Build history of the part. All positions in model axes, mm. Face numbers are marked on the shaded views. A direction names the side the tool comes from. Round coordinates to 2 decimals unless told otherwise and drop trailing zeros. Write each loop counter-clockwise with the first axis right and the second up, starting at its lowest first coordinate (ties: lowest second). Pieces come first, ordered by that corner, then holes. Notation, with made-up numbers: M 6,75 L 21,75 A19 cw 21,101 Z; hole C 43,51.5 d5. An arc over 180 degrees is marked long. Write item = value, one per line. Start each with the question number.
Q1. Drop flat-ended pins along their axis: P1, Ø10, axis at x = -36, z = 11, coming from the -Y side; P2, Ø16, axis at x = -37.5, z = 17, coming from the +Y side; P3, Ø3, axis at y = 9.5, z = 31.5, coming from the +X side; P4, Ø3, axis at y = 14, z = 18.5, coming from the -X side. Give the stop position or say it passes through.
Q2. Pull direction X, two halves, no side cores. Call the marked faces 6, 7 and 8: released by +X, released by -X, zero draft, split by the parting line, or undercut.
Q3. Band-saw the part on C-C on y = 29. Write the cut outline in (x, z).
Q4. Band-saw the part on B-B on x = -9.25. Write the cut outline in (y, z).
Q5. Probe L1, parallel to Y at x = -9, z = 2; L2, parallel to X at y = 11, z = 1.8; L3, parallel to Y at x = 14.5, z = 0.8. List the from-to ranges inside material, lowest first.
Q6. Tool access for the marked faces 1, 2, 3, 4 and 5: list every direction of +Z, -Z, +X, -X, +Y, -Y with a clear straight run to the whole face (end or side of a thin tool).
Q7. Band-saw the part on A-A on y = 9.5. Write the cut outline in (x, z), plus the area to 3 significant figures.
Q8. Band-saw the part on D-D on z = 13. Write the cut outline in (x, y), plus the area to 3 significant figures.
Autodesk Fusion 360 part; units mm, degrees
sketch "Szkic1" plane through (0, 0, 0) normal (0, 0, 1) x (1, 0, 0)
  line L0 (-20, 15) -> (1.5, 15)
  line L1 (1.5, 15) -> (1.5, 5)
  line L2 (1.5, 5) -> (-20, 5)
  line L3 (-20, 5) -> (-20, 15)
  line L4 (-23, 18) -> (4.5, 18)
  line L5 (4.5, 18) -> (4.5, 2)
  line L6 (4.5, 2) -> (-23, 2)
  line L7 (-23, 2) -> (-23, 18)
  line L8 (-43, 18) -> (24.5, 18)
  line L9 (24.5, 18) -> (24.5, 2)
  line L10 (24.5, 2) -> (-43, 2)
  line L11 (-43, 2) -> (-43, 18)
  line L12 (-23, 18) -> (4, 18)
  line L13 (4, 18) -> (4, 38)
  line L14 (4, 38) -> (-23, 38)
  line L15 (-23, 38) -> (-23, 18)
  dimension "d1" = 21.5
  dimension "d2" = 10
  dimension "d3" = 3
  dimension "d4" = 3
  dimension "d5" = 3
  dimension "d6" = 3
  dimension "d7" = 20
  dimension "d8" = 20
extrude "Wyciągnięcie proste4" add sketch "Szkic1" along normal blind 3 contours L4 L8 L12 L13 L14 L15 | L7 L8 L10 L11 | L5 L8 L9 L10 makes body 1 at (-36.3333, 12.6667, 0) makes body 2 at (17.8333, 7.3333, 0)
extrude "Wyciągnięcie proste5" add sketch "Szkic1" along normal blind 30 contours L4 L5 L6 L7 L8 L10 L12 bodies 1 2
extrude "Extrude6" add 1 faces at (-12.8333, 3, 30) along direction (0, 0, 1) blind 10 on bodies 1 bodies 1
extrude "Extrude7" add 1 faces at (-12.8333, 3, 40) along direction (0, 0, 1) blind 3 on bodies 1 bodies 1
sketch "Sketch2" plane through (0, 0, 0) normal (0, 1, 0) x (1, 0, 0)
  line L0 (-43, -3) -> (-23, -23)
  line L1 (-23, -23) -> (-23, -3)
  line L2 (-23, -3) -> (-43, -3)
  line L3 (24.5, -3) -> (4.5, -23)
  line L4 (4.5, -23) -> (4.5, -3)
  line L5 (4.5, -3) -> (24.5, -3)
  dimension "d23" = 135
extrude "Extrude8" add sketch "Sketch2" along normal blind 2 from surface at 2 contours L0 L1 L2 bodies 1
extrude "Extrude9" add sketch "Sketch2" along normal blind 2 from surface at 2 contours L3 L4 L5 bodies 1
extrude "Extrude10" add 1 faces at (4, 24.6667, 1) along direction (1, 0, 0) blind 0.5 on bodies 1 bodies 1
extrude "Extrude11" add 1 faces at (11.1667, 18, 1) along direction (0, 1, 0) blind 2 on bodies 1 bodies 1
extrude "Extrude12" add sketch "Sketch2" along normal blind 2 from surface at 18 contours L3 L4 L5 bodies 1
extrude "Extrude13" add sketch "Sketch2" along normal blind 2 from surface at 18 separate body contours L0 L1 L2 makes body 3
extrude "Extrude14" add 1 faces at (-36.3333, 18, 1) along direction (0, 1, 0) blind 2 on bodies 1 bodies 1 3
extrude "Extrude15" add 1 faces at (-13.8333, 18, 16.3333) along direction (0, 1, 0) blind 2 on bodies 1 bodies 1
sketch "Sketch3" plane through (4.5, 0, 0) normal (1, 0, 0) x (0, 1, 0)
  line L0 (20, 3) -> (20, 0)
  line L1 (20, 0) -> (38, 0)
  line L2 (38, 0) -> (38, 3)
  line L3 (38, 3) -> (20, 3)
  line L4 (20, 23) -> (38, 3)
  line L5 (20, 3) -> (20, 23)
sketch "Sketch4" plane through (-23, 0, 0) normal (-1, 0, 0) x (0, -1, 0)
  line L0 (-20, 0) -> (-20, 3)
  line L1 (-20, 3) -> (-38, 3)
  line L2 (-38, 3) -> (-38, 0)
  line L3 (-38, 0) -> (-20, 0)
  line L4 (-38, 3) -> (-20, 3)
  line L5 (-20, 23) -> (-38, 3)
  line L6 (-20, 23) -> (-20, 3)
extrude "Extrude16" add sketch "Sketch3" against normal blind 2 contours L3 L4 L5 bodies 1
extrude "Extrude17" add sketch "Sketch4" against normal blind 2 contours L1 L4 L5 L6 bodies 1
sketch "Sketch5" plane through (0, 0, 3) normal (0, 0, 1) x (-1, 0, 0)
  line L0 (-24.5, -18) -> (-4.5, -18)
  line L1 (-4.5, -18) -> (-4.5, -4)
  line L2 (-4.5, -4) -> (-24.5, -4)
  line L3 (-24.5, -4) -> (-24.5, -18)
  circle A0 centre (-14.5, -11) radius 2.5
  circle A1 centre (33, -11) radius 2.5
  line L4 (23, -2) -> (23, -20)
  circle A2 centre (9.25, -29) radius 2.5
  line L5 (21, -38) -> (21, -20)
  line L6 (21, -38) -> (-2.5, -38)
  dimension "d48" = 5
  dimension "d49" = 7
  dimension "d50" = 5
  dimension "d51" = 10
  dimension "d52" = 10
  dimension "d53" = 5
  dimension "d54" = 11.75
  dimension "d55" = 9
extrude "Extrude18" cut sketch "Sketch5" against normal blind 8 contours A0 | A1 | A2 bodies 1
equation "d23 = 180 deg - 45 deg"
equation "d34 = 14.00 mm + 4 mm"
equation "d37 = 14.00 mm + 4 mm"
equation "d54 = ( 23.5 / 2 ) * 1 mm"
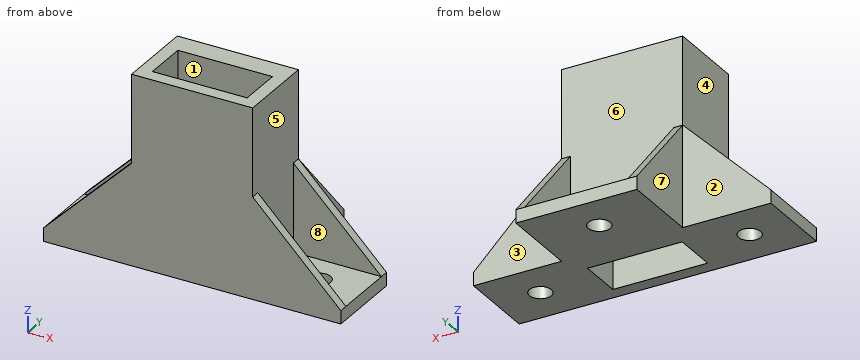
Conclusion:
q1.P1 = 2
q1.P2 = 20
q1.P3 = 4.5
q1.P4 = -23
q2.face_6 = undercut
q2.face_7 = released by -X
q2.face_8 = zero draft
q3.outline = M -23,0 L -11.75,0 L -11.75,3 L -21,3 L -21,13 L -23,13 Z; M -6.75,0 L 4.5,0 L 4.5,13 L 2.5,13 L 2.5,3 L -6.75,3 Z
q4.outline = M 2,0 L 5,0 L 5,43 L 2,43 Z; M 15,0 L 26.5,0 L 26.5,3 L 20,3 L 20,43 L 15,43 Z; M 31.5,0 L 38,0 L 38,3 L 31.5,3 Z
q5.L1 = 2 to 5, 15 to 26.51, 31.49 to 38
q5.L2 = -43 to -35.5, -30.5 to -20, 1.5 to 12, 17 to 24.5
q5.L3 = 2 to 8.5, 13.5 to 20
q6.face_1 = +Z, -Z
q6.face_2 = +Z, -Z, -X, +Y
q6.face_3 = +Z, -Z, +X, +Y
q6.face_4 = +Z, -X
q6.face_5 = +Z, +X
q7.outline = M -43,0 L -35,0 L -35,3 L -43,3 Z; M -31,0 L -20,0 L -20,43 L -23,43 L -23,3 L -31,3 Z; M 1.5,0 L 12.5,0 L 12.5,3 L 4.5,3 L 4.5,43 L 1.5,43 Z; M 16.5,0 L 24.5,0 L 24.5,3 L 16.5,3 Z
q7.area = 354 mm^2
q8.outline = M -33,2 L 14.5,2 L 14.5,4 L 4.5,4 L 4.5,18 L 14.5,18 L 14.5,20 L 4.5,20 L 4.5,29 L 2.5,29 L 2.5,20 L -21,20 L -21,29 L -23,29 L -23,20 L -33,20 L -33,18 L -23,18 L -23,4 L -33,4 Z; hole M -20,5 L 1.5,5 L 1.5,15 L -20,15 Z
q8.area = 396 mm^2
